```python
from build123d import *

# Parameters (mm, degrees)
F0_W     = 76.2
F0_H     = 50.8
F0_W_2   = 66.6496
F0_H_2   = 41.2496
F1_DEPTH = 304.8
F2_R     = 4.7752
F3_R     = 3.175


with BuildPart() as f1:
    # F0 (on Front) → F1 (new body)
    with BuildSketch(Plane.XZ):
        Rectangle(F0_W, F0_H)
        Rectangle(F0_W_2, F0_H_2, mode=Mode.SUBTRACT)
    extrude(amount=F1_DEPTH)

    # F2
    f2_edges = [f1.edges().sort_by_distance(p)[0] for p in [
        (38.1, -152.4, -25.4),
        (-38.1, -152.4, -25.4),
        (-38.1, -152.4, 25.4),
        (38.1, -152.4, 25.4),
    ]]
    fillet(f2_edges, radius=F2_R)

    # F3
    f3_edges = [f1.edges().sort_by_distance(p)[0] for p in [
        (-33.3248, -152.4, 20.6248),
        (33.3248, -152.4, 20.6248),
        (-33.3248, -152.4, -20.6248),
        (33.3248, -152.4, -20.6248),
    ]]
    fillet(f3_edges, radius=F3_R)


solid = f1.part
```
Check sheet for the modelled part. Datum: model origin and axes. Units: mm. A direction names the side the tool comes from. Give positions to 0.01 mm unless a question says otherwise; leave off trailing zeros. Order: outer loops, then holes, each group sorted by start corner. A loop starts at its lowest first (then second) coordinate and runs counter-clockwise, first axis right, second up. Notation, with made-up numbers: (72.5, 68.5) -> (76.5, 68.5) arc R36 ccw to (76.5, 102.5) -> close; hole circle Ø1 at (-26.75, -11). An arc over 180 degrees is marked (long way). Use CSV: the item, a comma, the result in double quotes. Start each with the question number.
1) Material ranges on line 1 (Z direction, x = 16, y = -71.5); line 2 (X direction, y = -227.5, z = -11); line 3 (X direction, y = -113, z = -20), recorded low to high. Write a range as from..to.
2) Set-up check for faces 1 (the face through (-36.7, -154.5, 24)), 2 (the face through (33.325, -150, 0)): record each of +Z, -Z, +X, -X, +Y, -Y from which the full face is reachable in a straight line by a thin tool's end or side.
3) Go/stop test with a flat-tipped pin: P1, Ø10, axis at x = 15, z = -18.5, coming from the +Y side. Record where the tip stops, or that it passes through.
4) Mould release check, pull along Z, two halves, no side actions. Record for faces 3 (the face through (-36.7, -154.5, -24)), 4 (the face through (0, -150, 20.625)), 5 (the face through (-1, 0, -22)): released by +Z, released by -Z, zero draft, split by the parting line, or undercut.
5) Sectioned sample at A-A, the plane z = 7. Record the boundary of the cut face in (x, y).
6) Sectioned sample at B-B, the plane x = -20. Record the boundary of the cut face in (y, z), plus the area to 3 significant figures.
7) Sectioned sample at C-C, the plane y = -65.5. Record the boundary of the cut face in (x, z) (3 decimals), plus the area to 3 significant figures.
Recorded:
1,line 1,"-25.4..-20.62, 20.62..25.4"
1,line 2,"-38.1..-33.32, 33.32..38.1"
1,line 3,"-38.1..-32.04, 32.04..38.1"
2,face 1,"+Z, -X, +Y, -Y"
2,face 2,"+Y, -Y"
3,P1,"y = 0"
4,face 3,"released by -Z"
4,face 4,"undercut"
4,face 5,"zero draft"
5,outline,"(-38.1, -304.8) -> (-33.32, -304.8) -> (-33.32, 0) -> (-38.1, 0) -> close; (33.32, -304.8) -> (38.1, -304.8) -> (38.1, 0) -> (33.32, 0) -> close"
6,outline,"(-304.8, -25.4) -> (0, -25.4) -> (0, -20.62) -> (-304.8, -20.62) -> close; (-304.8, 20.62) -> (0, 20.62) -> (0, 25.4) -> (-304.8, 25.4) -> close"
6,area,"2,910 mm2"
7,outline,"(-38.1, -20.625) arc R4.775 ccw to (-33.325, -25.4) -> (33.325, -25.4) arc R4.775 ccw to (38.1, -20.625) -> (38.1, 20.625) arc R4.775 ccw to (33.325, 25.4) -> (-33.325, 25.4) arc R4.775 ccw to (-38.1, 20.625) -> close; hole (-33.325, -17.45) arc R3.175 ccw to (-30.15, -20.625) -> (30.15, -20.625) arc R3.175 ccw to (33.325, -17.45) -> (33.325, 17.45) arc R3.175 ccw to (30.15, 20.625) -> (-30.15, 20.625) arc R3.175 ccw to (-33.325, 17.45) -> close"
7,area,"1,110 mm2"
